Read the model definition and answer for the solid it produces. Units are mm, in the model's axes. Give positions to 0.01 mm unless a question says otherwise; leave off trailing zeros. Write each loop counter-clockwise with the first axis right and the second up, starting at its lowest first coordinate (ties: lowest second). Pieces come first, ordered by that corner, then holes. Notation, with made-up numbers: M -2,40.5 L 48,40.5 A23 cw 48,67.5 Z; hole C 77,-28.5 d2. An arc over 180 degrees is marked long. Use a Markdown table: item, result. Add a question column.
Item 1: Consider probe 1 along Y at (x, z) = (233, 3); probe 2 along X at (y, z) = (106.5, 2.25) (3 decimals); probe 3 along X at (y, z) = (276, 4). Determine where each line is inside the solid, lowest interval first. Write a range as [from, to].
Item 2: A cutting plane is placed at A-A on x = 619. Determine the outline of the cut face in (y, z).
Item 3: A cutting plane is placed at D-D on x = 79. Determine the outline of the cut face in (y, z) (3 decimals).
Item 4: Given P1, Ø3, axis at x = 863.5, z = 4, coming from the -Y side (3 decimals); P2, Ø2, axis at x = 561, z = 1.5, coming from the -Y side; P3, Ø1.9, axis at y = 9, z = 3.5, coming from the -X side (3 decimals); P4, Ø1.9, axis at x = 48, z = 3, coming from the +Y side (3 decimals), each flat-ended and moving along its own axis, determine where each tip first touches the part or whether it passes through.
Item 5: A cutting plane is placed at B-B on y = 628.65. Determine the outline of the cut face in (x, z) (3 decimals), then the cut area to 3 significant figures.
Item 6: A cutting plane is placed at C-C on z = 4.25. Determine the outline of the cut face in (x, y) (3 decimals).
Autodesk Inventor part; units mm, degrees
ref_plane "YZ Plane" through (0, 0, 0) normal (1, 0, 0) x (0, 1, 0)
ref_plane "XZ Plane" through (0, 0, 0) normal (0, 1, 0) x (-1, 0, 0)
ref_plane "XY Plane" through (0, 0, 0) normal (0, 0, 1) x (1, 0, 0)
sketch "Sketch1" plane through (0, 0, 0) normal (0, 0, 1) x (1, 0, 0)
  line L0 (0, 0) -> (168.275, 0) construction
  line L1 (939.8, 0) -> (939.8, 168.275) construction
  line L2 (939.8, 685.8) -> (771.525, 685.8) construction
  line L3 (0, 685.8) -> (0, 517.525) construction
  line L4 (168.275, 517.525) -> (771.525, 517.525) construction
  line L5 (771.525, 517.525) -> (771.525, 168.275) construction
  line L6 (771.525, 168.275) -> (168.275, 168.275) construction
  line L7 (168.275, 168.275) -> (168.275, 517.525) construction
  line L8 (168.275, 517.525) -> (168.275, 685.8)
  line L9 (168.275, 517.525) -> (0, 517.525)
  line L10 (771.525, 517.525) -> (771.525, 685.8)
  line L11 (771.525, 517.525) -> (939.8, 517.525)
  line L12 (771.525, 168.275) -> (939.8, 168.275)
  line L13 (771.525, 168.275) -> (771.525, 0)
  line L14 (168.275, 168.275) -> (168.275, 0)
  line L15 (168.275, 168.275) -> (0, 168.275)
  line L16 (771.525, 685.8) -> (168.275, 685.8)
  line L17 (168.275, 685.8) -> (0, 685.8) construction
  line L18 (939.8, 517.525) -> (939.8, 685.8) construction
  line L19 (168.275, 0) -> (393.7, 0)
  line L20 (771.525, 0) -> (939.8, 0) construction
  line L21 (0, 168.275) -> (0, 0) construction
  line L22 (0, 517.525) -> (0, 168.275)
  line L23 (939.8, 168.275) -> (939.8, 517.525)
  line L24 (393.7, 0) -> (393.7, 25.4)
  line L25 (546.1, 0) -> (546.1, 25.4)
  line L26 (393.7, 25.4) -> (215.9, 25.4)
  line L27 (292.1, 203.2) -> (292.1, 279.4)
  line L28 (647.7, 279.4) -> (647.7, 25.4)
  line L29 (647.7, 25.4) -> (546.1, 25.4)
  line L30 (546.1, 0) -> (771.525, 0)
  line L31 (393.7, 0) -> (546.1, 0) construction
  line L32 (450.85, 279.4) -> (450.85, 304.8)
  line L33 (450.85, 304.8) -> (488.95, 304.8)
  line L34 (488.95, 304.8) -> (488.95, 279.4)
  line L35 (292.1, 279.4) -> (450.85, 279.4)
  line L36 (488.95, 279.4) -> (647.7, 279.4)
  circle A0 centre (469.9, 628.65) radius 25.4
  line L37 (292.1, 203.2) -> (215.9, 203.2)
  line L38 (215.9, 203.2) -> (215.9, 25.4)
  point P0 (469.9, 685.8)
  dimension "d0" = 939.8
  dimension "d1" = 685.8
  dimension "d2" = 603.25
  dimension "d3" = 349.25
  dimension "d4" = 168.275
  dimension "d5" = 168.275
  dimension "d6" = 168.275
  dimension "d8" = 168.275
  dimension "d11" = 152.4
  dimension "d12" = 225.425
  dimension "d13" = 225.425
  dimension "d14" = 25.4
  dimension "d15" = 355.6
  dimension "d17" = 25.4
  dimension "d18" = 38.1
  dimension "d19" = 50.8
  dimension "d20" = 57.15
  dimension "d21" = 254
  dimension "d22" = 123.825
  dimension "d23" = 123.825
  dimension "d24" = 76.2
  dimension "d25" = 177.8
extrude "Extrusion1" add sketch "Sketch1" along normal blind 6.35
equation "\"d4\" = d6"
equation "\"d5\" = d8"
equation "\"d12\" = d13"
equation "\"d22\" = d23"
properties part number "belly pan"
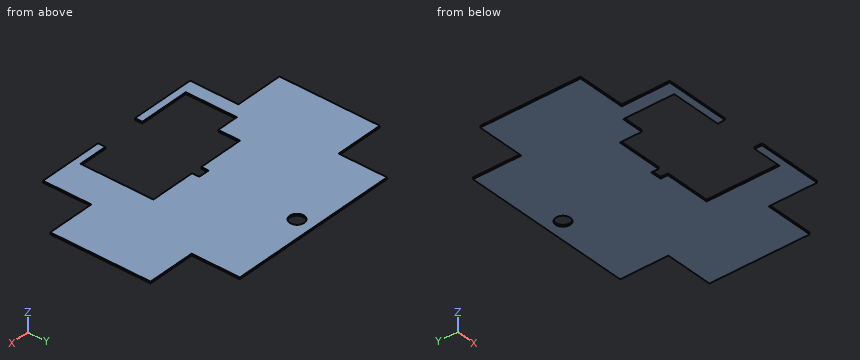
Filled in:
| question | item | result |
|---|---|---|
| 1 | probe 1 | [0, 25.4], [203.2, 685.8] |
| 1 | probe 2 | [168.275, 215.9], [647.7, 771.525] |
| 1 | probe 3 | [0, 292.1], [647.7, 939.8] |
| 2 | outline | M 0,0 L 25.4,0 L 25.4,6.35 L 0,6.35 Z; M 279.4,0 L 685.8,0 L 685.8,6.35 L 279.4,6.35 Z |
| 3 | outline | M 168.275,0 L 517.525,0 L 517.525,6.35 L 168.275,6.35 Z |
| 4 | P1 | y = 168.275 |
| 4 | P2 | y = 0 |
| 4 | P3 | x = 168.275 |
| 4 | P4 | y = 517.525 |
| 5 | outline | M 168.275,0 L 444.5,0 L 444.5,6.35 L 168.275,6.35 Z; M 495.3,0 L 771.525,0 L 771.525,6.35 L 495.3,6.35 Z |
| 5 | area | 3,510 mm² |
| 6 | outline | M 0,168.275 L 168.275,168.275 L 168.275,0 L 393.7,0 L 393.7,25.4 L 215.9,25.4 L 215.9,203.2 L 292.1,203.2 L 292.1,279.4 L 450.85,279.4 L 450.85,304.8 L 488.95,304.8 L 488.95,279.4 L 647.7,279.4 L 647.7,25.4 L 546.1,25.4 L 546.1,0 L 771.525,0 L 771.525,168.275 L 939.8,168.275 L 939.8,517.525 L 771.525,517.525 L 771.525,685.8 L 168.275,685.8 L 168.275,517.525 L 0,517.525 Z; hole C 469.9,628.65 d50.8 |
